Verification items for the finished model (mm, model axes). A direction names the side the tool comes from. Give positions to 0.01 mm unless a question says otherwise; leave off trailing zeros. Loops run counter-clockwise (first coordinate to the right, second up) from the corner with the lowest first, then second, coordinate; pieces in that order, holes last. Notation, with made-up numbers: (77, 62) - (129, 62) arc R20 cw to (129, 83) - close; hole circle Ø5 at (-31.75, 6). An arc over 180 degrees is marked (long way). Use one line per item in the form item = value.
```python
from build123d import *

# Parameters (mm, degrees)
SKETCH_1_W          = 775
SKETCH_1_H          = 75
EXTRUDE_1_DEPTH     = 3
EXTRUDE_START       = -3
SKETCH_2_W          = 775
SKETCH_2_H          = 3
EXTRUDE_2_DEPTH     = 20
SKETCH_3_R          = 3.25
CUT_EXTRUDE_1_DEPTH = 779.806137623
FILLET_1_R          = 5
SKETCH_4_R          = 2.5
CUT_EXTRUDE_2_DEPTH = 779.594246061
FILLET_2_R          = 2


with BuildPart() as part:
    # 스케치1 → 보스-돌출1 (new body)
    with BuildSketch(Plane.XY):
        with Locations((387.5, 37.5)):
            Rectangle(SKETCH_1_W, SKETCH_1_H)
    extrude(amount=EXTRUDE_1_DEPTH)

    # 스케치2 → 보스-돌출2 (add)
    with BuildSketch(Plane.XY.offset(3).offset(EXTRUDE_START)):
        with Locations((387.5, 1.5)):
            Rectangle(SKETCH_2_W, SKETCH_2_H)
    extrude(amount=EXTRUDE_2_DEPTH)

    # 스케치3 → 컷-돌출1 (cut, through all)
    with BuildSketch(Plane.XY.offset(3)):
        with Locations((107.5, 55)):
            Circle(SKETCH_3_R)
        with Locations((107.5, 20)):
            Circle(SKETCH_3_R)
        with Locations((387.5, 55)):
            Circle(SKETCH_3_R)
        with Locations((387.5, 20)):
            Circle(SKETCH_3_R)
        with Locations((667.5, 55)):
            Circle(SKETCH_3_R)
        with Locations((667.5, 20)):
            Circle(SKETCH_3_R)
    extrude(amount=-CUT_EXTRUDE_1_DEPTH, mode=Mode.SUBTRACT)

    # 필렛1
    fillet_1_edges = [part.edges().sort_by_distance(p)[0] for p in [
        (387.5, 0, 0),
    ]]
    fillet(fillet_1_edges, radius=FILLET_1_R)

    # 스케치4 → 컷-돌출2 (cut, through all)
    with BuildSketch(Plane(origin=(0, 3, 0), x_dir=(1, 0, 0), z_dir=(0, 1, 0))):
        with Locations(Location((60, -11.5, 0), (0, 0, 270))):
            Circle(SKETCH_4_R)
        with Locations(Location((715, -11.5, 0), (0, 0, 270))):
            Circle(SKETCH_4_R)
    extrude(amount=-CUT_EXTRUDE_2_DEPTH, mode=Mode.SUBTRACT)

    # 필렛2
    fillet_2_edges = [part.edges().sort_by_distance(p)[0] for p in [
        (387.5, 3, 3),
    ]]
    fillet(fillet_2_edges, radius=FILLET_2_R)


solid = part.part
```
1. Scan lines: probe 1 along Y at (x, z) = (667.5, 0.95); probe 2 along Y at (x, z) = (107.5, 2.35); probe 3 along Y at (x, z) = (203.5, 6.25). Record each from-to range of solid material in increasing order.
Result set:
probe_1 = 2.07 to 16.75, 23.25 to 51.75, 58.25 to 75
probe_2 = 0.76 to 16.75, 23.25 to 51.75, 58.25 to 75
probe_3 = 0 to 3
2. Section check B-B, the plane y = 42. Record the cut outline in (x, z), then the cut area to 4 significant figures.
Result set:
outline = (0, 0) - (775, 0) - (775, 3) - (0, 3) - close
area = 2,325 mm²
3. Section check A-A, the plane x = 346. Record the cut outline in (y, z).
Result set:
outline = (0, 5) arc R5 ccw to (5, 0) - (75, 0) - (75, 3) - (5, 3) arc R2 cw to (3, 5) - (3, 20) - (0, 20) - close
4. Tool access check on faces 1 (the flat face through (382, 3, 12)), 2 (the flat face through (382, 0, 12)). Record the directions out of +Z, -Z, +X, -X, +Y, -Y that give a thin tool (end or side, any length) a straight path to the whole face; none if there is none.
Result set:
face_1 = +Z, +X, -X, +Y
face_2 = +Z, -Z, +X, -X, -Y
5. Depth check by flat-ended pin: pin 1 Ø2 at (x, z) = (403, 17) entering from +Y; pin 2 Ø4.5 at (x, z) = (715, 11.5) entering from -Y; pin 3 Ø8.5 at (x, y) = (107.5, 55) entering from +Z; pin 4 Ø4 at (x, y) = (659, 30.5) entering from -Z. Enter the tip coordinate at first touch or a pass-through.
Result set:
pin_1 = 3
pin_2 = through
pin_3 = 3
pin_4 = 0
